Geometry check sheet. Reference: drawing and pictorial views, mm from the part's lowest x, y, z. A direction names the side the tool comes from. Coordinates: 2 decimals unless noted, no trailing zeros. Loops run counter-clockwise (first coordinate to the right, second up) from the corner with the lowest first, then second, coordinate; pieces in that order, holes last.
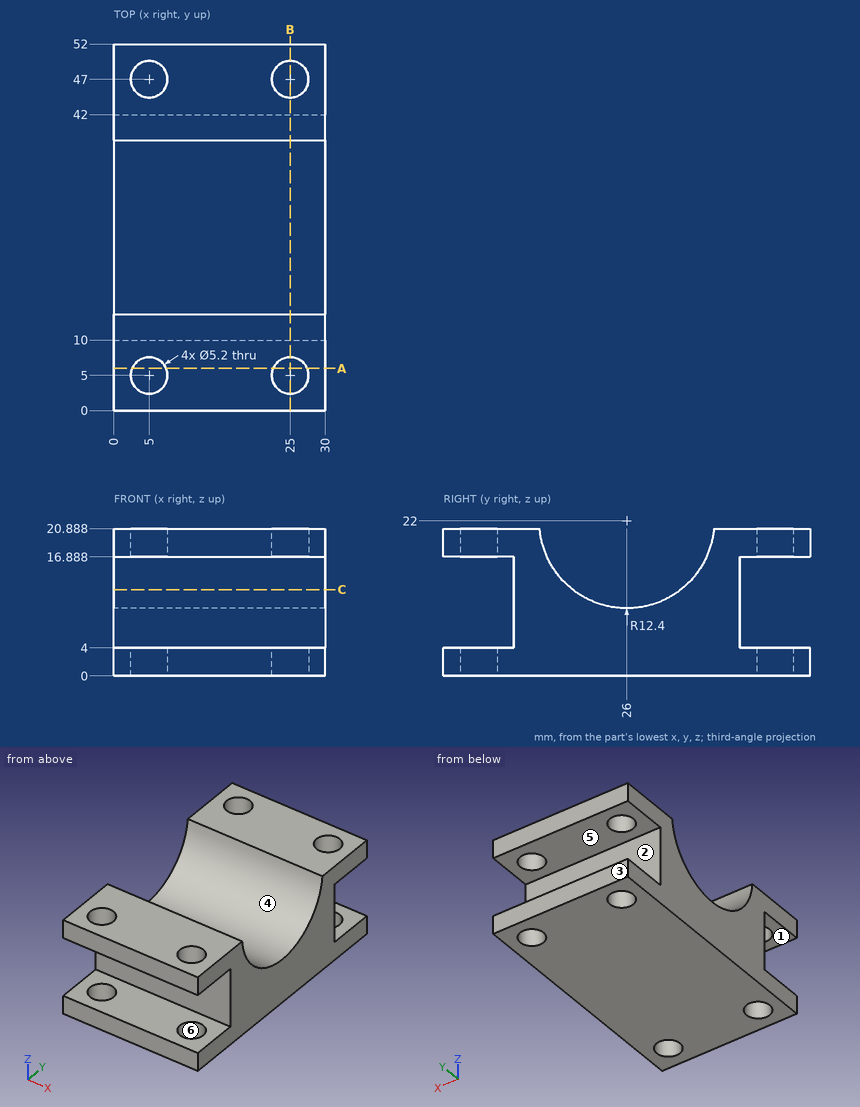
1) Section check B-B on x = 25. Count the separate pieces of the cut face and the enclosed holes in it, and give its area (3 significant figures).
Data:
separate pieces: 5
enclosed holes: 0
area: 531 mm2
2) Section check C-C on z = 12.25. Record the cut outline in (x, y), and give its area (3 significant figures).
Data:
outline: (0, 10) - (30, 10) - (30, 18.34) - (0, 18.34) - close; (0, 33.66) - (30, 33.66) - (30, 42) - (0, 42) - close
area: 500 mm2
3) Access from +Z, -Z, +X, -X, +Y, -Y to the whole of each face (thin tool, end or side, straight path). Record for the marked faces 1, 2 and 3.
Data:
face 1: +X, -X, -Y
face 2: +X, -X, +Y
face 3: +Z, -Z, +X, -X, +Y
4) Section check A-A on y = 6. Record the cut outline in (x, z), and give its area (3 significant figures).
Data:
outline: (0, 0) - (2.6, 0) - (2.6, 4) - (0, 4) - close; (0, 16.89) - (2.6, 16.89) - (2.6, 20.89) - (0, 20.89) - close; (7.4, 0) - (22.6, 0) - (22.6, 4) - (7.4, 4) - close; (7.4, 16.89) - (22.6, 16.89) - (22.6, 20.89) - (7.4, 20.89) - close; (27.4, 0) - (30, 0) - (30, 4) - (27.4, 4) - close; (27.4, 16.89) - (30, 16.89) - (30, 20.89) - (27.4, 20.89) - close
area: 163 mm2
5) Mould release check, pull along Z, two halves, no side actions. Record for the marked faces 4, 5 and 6: +Z half, -Z half, draft (parallel to the pull), parting line (faces both ways), or undercut.
Data:
face 4: +Z half
face 5: undercut
face 6: draft
6) Material ranges on probe 1 along X at (y, z) = (5, 19.55); probe 2 along Y at (x, z) = (5, 0.95); probe 3 along X at (y, z) = (49, 17.25), recorded low to high.
Data:
probe 1: x = 0 to 2.4, 7.6 to 22.4, 27.6 to 30
probe 2: y = 0 to 2.4, 7.6 to 44.4, 49.6 to 52
probe 3: x = 0 to 3.34, 6.66 to 23.34, 26.66 to 30
7) Depth check by flat-ended pin: pin 1 (8.5 mm diameter, centred on x = 5, y = 47, fed in from -Z); pin 2 (1.5 mm diameter, centred on x = 24, y = 34, fed in from +Z) (1 decimal); pin 3 (6.5 mm diameter, centred on x = 7.5, z = 8, fed in from -Y); pin 4 (10 mm diameter, centred on x = 7.5, y = 20.5, fed in from +Z) (1 decimal). Enter the tip coordinate at first touch or a pass-through.
Data:
pin 1: stops at z = 0
pin 2: stops at z = 13.2
pin 3: stops at y = 10
pin 4: stops at z = 15.4
